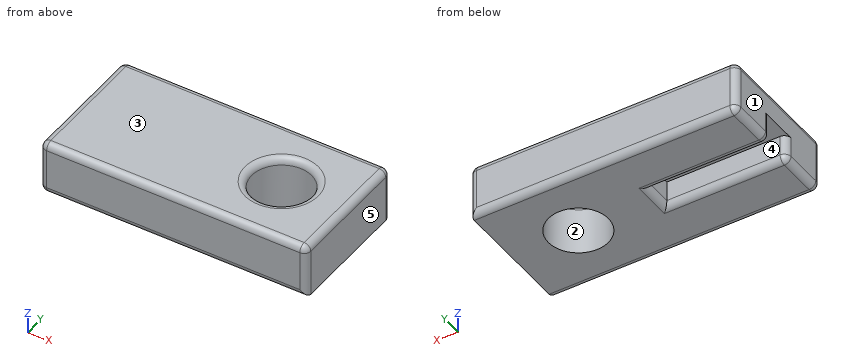
```python
from build123d import *

# Parameters (mm, degrees)
F0_R         = 2.25
F1_DEPTH     = 4
F2_W         = 9
F2_H         = 3
F3_DEPTH     = 2
F4_R         = 0.5
F5_T1_DEPTH  = 8.5
F5_T3_DEPTH  = 2
F5_T5_DEPTH  = 2.9
F5_T7_DEPTH  = 2.9
F5_S11_W     = 0.5
F5_S11_H     = 0.5
F5_T12_DEPTH = 0.5
F5_S17_W     = 0.5
F5_S17_H     = 0.5
F5_T18_DEPTH = 0.5
F5_T22_ANGLE = 90
F5_T24_ANGLE = 90
F5_T29_DEPTH = 9.75
F5_T33_DEPTH = 3.25
F5_T40_DEPTH = 9.75
F5_T44_DEPTH = 3.25


# Not quite as in the source:
# - a fillet or chamfer that OpenCascade refuses, or shapes differently, is made with other operations: its cross-section is extruded or revolved along the edge and cut away or added


with BuildPart() as f1:
    # F0 (on Top) → F1 (new body)
    with BuildSketch(Plane.XY):
        with BuildLine():
            Line((20, 0), (20, 9.8))
            Line((20, 9.8), (0, 9.8))
            Line((0, 9.8), (0, 6.4))
            ThreePointArc((0, 6.4), (0.1464466094, 6.0464466094), (0.5, 5.9))
            Line((0.5, 5.9), (9, 5.9))
            Line((9, 5.9), (9, 3.9))
            Line((9, 3.9), (0.5, 3.9))
            ThreePointArc((0.5, 3.9), (0.1464466094, 3.7535533906), (0, 3.4))
            Line((0, 3.4), (0, 0))
            Line((0, 0), (20, 0))
        make_face()
        with Locations((15, 4.9)):
            Circle(F0_R, mode=Mode.SUBTRACT)
    extrude(amount=F1_DEPTH)

    # F2 (on face) → F3 (join)
    with BuildSketch(Plane.XY.offset(4)):
        with Locations((4.5, 4.9)):
            Rectangle(F2_W, F2_H)
    extrude(amount=-F3_DEPTH)

    # F4
    f4_edges = [f1.edges().sort_by_distance(p)[0] for p in [
        (10, 0, 4),
        (20, 4.9, 4),
        (10, 9.8, 4),
        (0, 4.9, 4),
        (12.75, 4.9, 4),
        (20, 9.8, 2),
        (0, 9.8, 2),
        (10, 9.8, 0),
        (0, 0, 2),
        (20, 0, 2),
        (10, 0, 0),
    ]]
    fillet(f4_edges, radius=F4_R)

    # F5: fillet of radius 0.5 on 3 edges, made by hand

    # F5_s2 → F5_t1 (cut)
    with BuildSketch(Plane.YZ.offset(0.5)):
        with BuildLine():
            ThreePointArc((6.4, 0), (6.0464466094, 0.1464466094), (5.9, 0.5))
            Line((5.9, 0.5), (5.9, 0))
            Line((5.9, 0), (6.4, 0))
        make_face()
        with BuildLine():
            ThreePointArc((3.4, 0), (3.7535533906, 0.1464466094), (3.9, 0.5))
            Line((3.9, 0.5), (3.9, 0))
            Line((3.9, 0), (3.4, 0))
        make_face()
    extrude(amount=F5_T1_DEPTH, mode=Mode.SUBTRACT)

    # F5_s4 → F5_t3 (cut)
    with BuildSketch(Plane.XZ.offset(-5.9)):
        with BuildLine():
            ThreePointArc((9.5, 0), (9.1464466094, 0.1464466094), (9, 0.5))
            Line((9, 0.5), (9, 0))
            Line((9, 0), (9.5, 0))
        make_face()
    extrude(amount=F5_T3_DEPTH, mode=Mode.SUBTRACT)

    # F5_s6 → F5_t5 (cut)
    with BuildSketch(Plane.XZ.offset(-3.4)):
        with BuildLine():
            ThreePointArc((0.5, 0), (0.1464466094, 0.1464466094), (0, 0.5))
            Line((0, 0.5), (0, 0))
            Line((0, 0), (0.5, 0))
        make_face()
    extrude(amount=F5_T5_DEPTH, mode=Mode.SUBTRACT)

    # F5_s8 → F5_t7 (cut)
    with BuildSketch(Plane.XZ.offset(-9.3)):
        with BuildLine():
            ThreePointArc((0.5, 0), (0.1464466094, 0.1464466094), (0, 0.5))
            Line((0, 0.5), (0, 0))
            Line((0, 0), (0.5, 0))
        make_face()
    extrude(amount=F5_T7_DEPTH, mode=Mode.SUBTRACT)


with BuildPart() as f5_tool10:
    # F5_s11 → F5_t12 (new body)
    with BuildSketch(Plane.XY.offset(0.5)):
        with Locations((0.25, 0.25)):
            Rectangle(F5_S11_W, F5_S11_H)
    extrude(amount=-F5_T12_DEPTH)

    # F5_s13 → F5_t14 (revolve, cut)
    with BuildSketch(Plane(origin=(0.5, 0.5, 0.5), x_dir=(0.7071067812, 0.7071067812, 0), z_dir=(-0.7071067812, 0.7071067812, 0))):
        with BuildLine():
            ThreePointArc((0, -0.5), (0.5, 0), (0, 0.5))
            Line((0, 0.5), (0, -0.5))
        make_face()
    revolve(axis=Axis((0.5, 0.5, 0.5), (0, 0, -1)), mode=Mode.SUBTRACT)


with BuildPart() as f1_1:
    add(f1.part)

    # F5_t9: cut F5_tool10
    add(f5_tool10.part, mode=Mode.SUBTRACT)


with BuildPart() as f5_tool16:
    # F5_s17 → F5_t18 (new body)
    with BuildSketch(Plane.XY.offset(0.5)):
        with Locations((0.25, 9.55)):
            Rectangle(F5_S17_W, F5_S17_H)
    extrude(amount=-F5_T18_DEPTH)

    # F5_s19 → F5_t20 (revolve, cut)
    with BuildSketch(Plane(origin=(0.5, 9.3, 0.5), x_dir=(0.7071067812, -0.7071067812, 0), z_dir=(0.7071067812, 0.7071067812, 0))):
        with BuildLine():
            ThreePointArc((0, -0.5), (0.5, 0), (0, 0.5))
            Line((0, 0.5), (0, -0.5))
        make_face()
    revolve(axis=Axis((0.5, 9.3, 0.5), (0, 0, -1)), mode=Mode.SUBTRACT)


with BuildPart() as f1_2:
    add(f1_1.part)

    # F5_t15: cut F5_tool16
    add(f5_tool16.part, mode=Mode.SUBTRACT)

    # F5_s21 → F5_t22 (revolve, cut)
    with BuildSketch(Plane.YZ.offset(0.5)):
        with BuildLine():
            ThreePointArc((3.4, 0), (3.7535533906, 0.1464466094), (3.9, 0.5))
            Line((3.9, 0.5), (3.9, 0))
            Line((3.9, 0), (3.4, 0))
        make_face()
    revolve(axis=Axis((0.5, 3.4, 0), (0, 0, 1)), revolution_arc=F5_T22_ANGLE, mode=Mode.SUBTRACT)

    # F5_s23 → F5_t24 (revolve, cut)
    with BuildSketch(Plane.XZ.offset(-6.4)):
        with BuildLine():
            ThreePointArc((0.5, 0), (0.1464466094, 0.1464466094), (0, 0.5))
            Line((0, 0.5), (0, 0))
            Line((0, 0), (0.5, 0))
        make_face()
    revolve(axis=Axis((0.5, 6.4, 0), (0, 0, 1)), revolution_arc=F5_T24_ANGLE, mode=Mode.SUBTRACT)


with BuildPart() as f5_tool27:
    # F5_s28 → F5_t29 (new body)
    with BuildSketch(Plane.YZ.offset(0.5)):
        with BuildLine():
            ThreePointArc((6.4, 0), (6.0464466094, 0.1464466094), (5.9, 0.5))
            Line((5.9, 0.5), (5.9, 0))
            Line((5.9, 0), (6.4, 0))
        make_face()
    extrude(amount=F5_T29_DEPTH)

    split(bisect_by=Plane.YZ.offset(9), keep=Keep.TOP)


with BuildPart() as f5_tool31:
    # F5_s32 → F5_t33 (new body)
    with BuildSketch(Plane.XZ.offset(-7.15)):
        with BuildLine():
            ThreePointArc((9.5, 0), (9.1464466094, 0.1464466094), (9, 0.5))
            Line((9, 0.5), (9, 0))
            Line((9, 0), (9.5, 0))
        make_face()
    extrude(amount=F5_T33_DEPTH)

    split(bisect_by=Plane.XZ.offset(-5.9), keep=Keep.BOTTOM)


with BuildPart() as f5_tool27_1:
    add(f5_tool27.part)

    # F5_t35: intersect F5_tool31
    add(f5_tool31.part, mode=Mode.INTERSECT)


with BuildPart() as f1_3:
    add(f1_2.part)

    # F5_t25: cut F5_tool27
    add(f5_tool27_1.part, mode=Mode.SUBTRACT)


with BuildPart() as f5_tool38:
    # F5_s39 → F5_t40 (new body)
    with BuildSketch(Plane.YZ.offset(10.25)):
        with BuildLine():
            ThreePointArc((3.4, 0), (3.7535533906, 0.1464466094), (3.9, 0.5))
            Line((3.9, 0.5), (3.9, 0))
            Line((3.9, 0), (3.4, 0))
        make_face()
    extrude(amount=-F5_T40_DEPTH)

    split(bisect_by=Plane.YZ.offset(9), keep=Keep.TOP)


with BuildPart() as f5_tool42:
    # F5_s43 → F5_t44 (new body)
    with BuildSketch(Plane.XZ.offset(-5.9)):
        with BuildLine():
            ThreePointArc((9.5, 0), (9.1464466094, 0.1464466094), (9, 0.5))
            Line((9, 0.5), (9, 0))
            Line((9, 0), (9.5, 0))
        make_face()
    extrude(amount=F5_T44_DEPTH)

    split(bisect_by=Plane.XZ.offset(-3.9), keep=Keep.TOP)


with BuildPart() as f5_tool38_1:
    add(f5_tool38.part)

    # F5_t46: intersect F5_tool42
    add(f5_tool42.part, mode=Mode.INTERSECT)


with BuildPart() as f1_4:
    add(f1_3.part)

    # F5_t36: cut F5_tool38
    add(f5_tool38_1.part, mode=Mode.SUBTRACT)


solid = f1_4.part
```
Geometry: final body of the model. Coordinates: model frame, mm. Face numbers are marked on the shaded views. A direction names the side the tool comes from. Give positions to 0.01 mm unless a question says otherwise; leave off trailing zeros. Write each loop counter-clockwise with the first axis right and the second up, starting at its lowest first coordinate (ties: lowest second). Pieces come first, ordered by that corner, then holes.
1. Section query D-D, the plane x = 8.75. Return loops of the section in (y, z), then the cut area to 3 significant figures.
2. Pin query (flat end, axial travel): P1, Ø2.5, axis at x = 6, y = 5, coming from the -Z side; P2, Ø1.6, axis at y = 5, z = 1, coming from the -X side; P3, Ø2, axis at x = 14.5, y = 7.5, coming from the +Z side. Return the tip coordinate at first contact, or that it passes through.
3. Line query: probe 1 along Y at (x, z) = (15, 2.35); probe 2 along Z at (x, y) = (8, 5.25); probe 3 along Y at (x, z) = (11, 3.55). Output: solid intervals per line, ascending.
4. Section query A-A, the plane y = 4.9. Return loops of the section in (x, z).
5. Section query C-C, the plane x = 15. Return loops of the section in (y, z), then the cut area to 3 significant figures.
6. Section query B-B, the plane z = 3. Return loops of the section in (x, y).
7. Reachability of the marked faces 4 and 5 from +Z, -Z, +X, -X, +Y, -Y: full face, straight path, thin tool, end or side. Return the list, or none.
8. Draft query along X for the marked faces 1, 2 and 3. Return one class per face: released by +X, released by -X, zero draft, split by the parting line, or undercut.
Computed:
1. outline: (0, 0.5) arc R0.5 ccw to (0.5, 0) - (3.4, 0) arc R0.5 ccw to (3.9, 0.5) - (3.9, 2) - (5.9, 2) - (5.9, 0.5) arc R0.5 ccw to (6.4, 0) - (9.3, 0) arc R0.5 ccw to (9.8, 0.5) - (9.8, 3.5) arc R0.5 ccw to (9.3, 4) - (0.5, 4) arc R0.5 ccw to (0, 3.5) - close
1. area: 34.9 mm2
2. P1: stops at z = 0.02
2. P2: stops at x = 9
2. P3: stops at z = 4
3. probe 1: y = 0 to 2.65, 7.15 to 9.8
3. probe 2: z = 2 to 4
3. probe 3: y = 0 to 9.8
4. outline: (0, 2) - (9, 2) - (9, 0.5) arc R0.5 ccw to (9.5, 0) - (12.75, 0) - (12.75, 3.5) arc R0.5 ccw to (12.25, 4) - (0.5, 4) arc R0.5 ccw to (0, 3.5) - close; (17.25, 0) - (20, 0) - (20, 3.5) arc R0.5 ccw to (19.5, 4) - (17.75, 4) arc R0.5 ccw to (17.25, 3.5) - close
5. outline: (0, 0.5) arc R0.5 ccw to (0.5, 0) - (2.65, 0) - (2.65, 3.5) arc R0.5 ccw to (2.15, 4) - (0.5, 4) arc R0.5 ccw to (0, 3.5) - close; (7.15, 0) - (9.3, 0) arc R0.5 ccw to (9.8, 0.5) - (9.8, 3.5) arc R0.5 ccw to (9.3, 4) - (7.65, 4) arc R0.5 ccw to (7.15, 3.5) - close
5. area: 20.9 mm2
6. outline: (0, 0.5) arc R0.5 ccw to (0.5, 0) - (19.5, 0) arc R0.5 ccw to (20, 0.5) - (20, 9.3) arc R0.5 ccw to (19.5, 9.8) - (0.5, 9.8) arc R0.5 ccw to (0, 9.3) - close; hole circle Ø4.5 at (15, 4.9)
7. face 4: -Z, -X
7. face 5: +Z, -Z, +X, +Y, -Y
8. face 1: released by -X
8. face 2: undercut
8. face 3: zero draft
